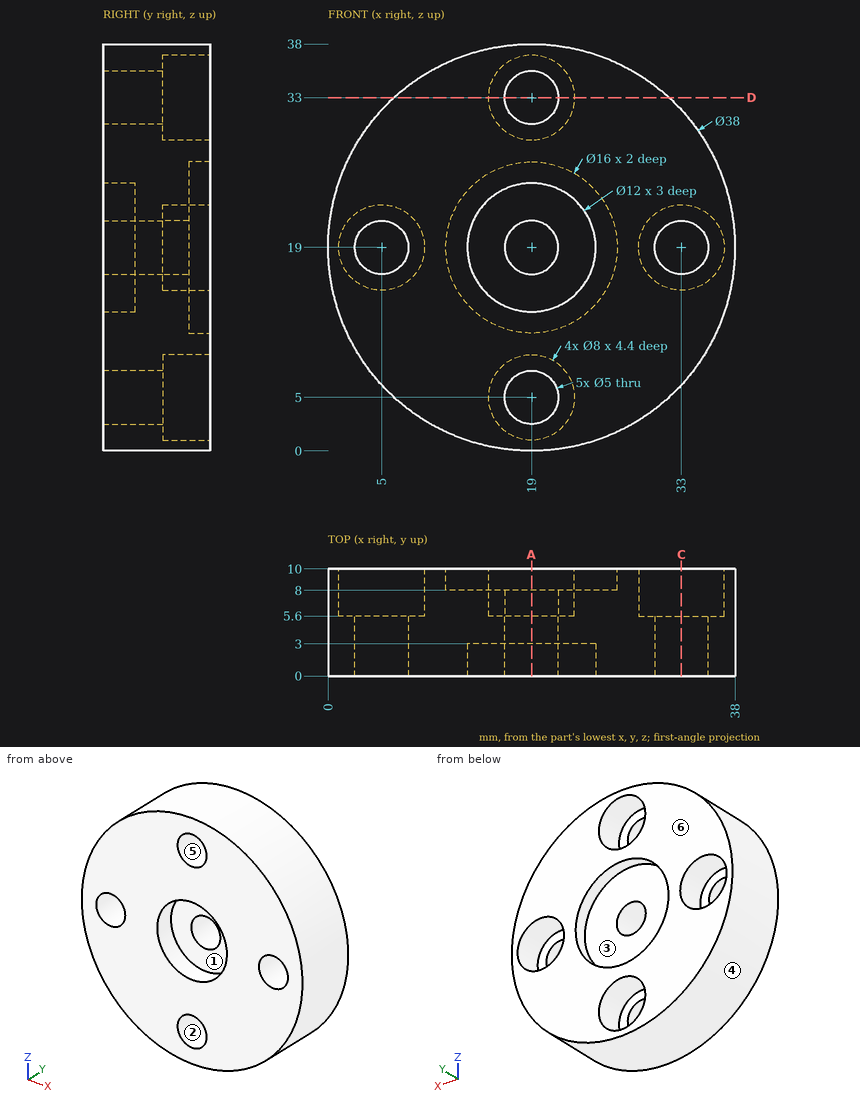
Geometry: see drawing. Coordinates: mm, zero at the bounding-box minimum. A direction names the side the tool comes from. Round coordinates to 2 decimals unless told otherwise and drop trailing zeros. Write each loop counter-clockwise with the first axis right and the second up, starting at its lowest first coordinate (ties: lowest second). Pieces come first, ordered by that corner, then holes. Notation, with made-up numbers: M -16.75,14 L -1.75,14 A18 cw -1.75,23 Z; hole C 77.5,52.25 d1. An arc over 180 degrees is marked long. Answer in a Markdown table with one row per item. Add a question column.
(1) Cut plane D-D, the plane z = 33. Return the cut outline in (x, y), then the cut area to 3 significant figures.
(2) Ray query, L1, parallel to Z at x = 19.5, y = 2.5; L2, parallel to X at y = 2.5, z = 20.5; L3, parallel to Y at x = 3.5, z = 16. Return the intervals inside material, ascending.
(3) Draft query along Z for the marked faces 4, 5 and 6. Return one class per face: pulls with the +Z half, pulls with the -Z half, needs draft (parallel to the pull), parting line crosses it, or undercut.
(4) Cut plane C-C, the plane x = 33. Return the cut outline in (y, z), then the cut area to 3 significant figures.
(5) Reachability of the marked faces 1, 2 and 3 from +Z, -Z, +X, -X, +Y, -Y: full face, straight path, thin tool, end or side. Return the list, or none.
(6) Cut plane A-A, the plane x = 19. Give the number of separate pieces and of enclosed holes in the cut face, then the cut area to 3 significant figures.
(7) Contact query for flat-ended pins moving along their axis: pin 1 (4.5 mm diameter, centred on x = 19, z = 19, fed in from -Y); pin 2 (7 mm diameter, centred on x = 19, z = 19, fed in from +Y); pin 3 (1 mm diameter, centred on x = 32.5, y = 6, fed in from -Z); pin 4 (4 mm diameter, centred on x = 17.5, z = 33.5, fed in from +Y). Output: stop coordinate, or through.
Established:
| question | item | result |
|---|---|---|
| 1 | outline | M 6.15,0 L 16.5,0 L 16.5,5.6 L 15,5.6 L 15,10 L 6.15,10 Z; M 21.5,0 L 31.85,0 L 31.85,10 L 23,10 L 23,5.6 L 21.5,5.6 Z |
| 1 | area | 194 mm² |
| 2 | L1 | 0.01 to 2.55, 7.45 to 13.02, 24.98 to 30.55, 35.45 to 37.99 |
| 2 | L2 | 0.06 to 3, 7 to 13.19, 24.81 to 31, 35 to 37.94 |
| 2 | L3 | 0 to 5.6 |
| 3 | face 4 | parting line crosses it |
| 3 | face 5 | undercut |
| 3 | face 6 | needs draft |
| 4 | outline | M 0,6.15 L 10,6.15 L 10,15 L 5.6,15 L 5.6,16.5 L 0,16.5 Z; M 0,21.5 L 5.6,21.5 L 5.6,23 L 10,23 L 10,31.85 L 0,31.85 Z |
| 4 | area | 194 mm² |
| 5 | face 1 | -Y |
| 5 | face 2 | +Y, -Y |
| 5 | face 3 | +Y |
| 6 | separate pieces | 4 |
| 6 | enclosed holes | 0 |
| 6 | area | 161 mm² |
| 7 | pin 1 | through |
| 7 | pin 2 | y = 8 |
| 7 | pin 3 | z = 5.14 |
| 7 | pin 4 | y = 5.6 |
